Part model, mm, in its own coordinate system. Face numbers are marked on the shaded views. Coordinates: 2 decimals unless noted, no trailing zeros. Order: outer loops, then holes, each group sorted by start corner. A loop starts at its lowest first (then second) coordinate and runs counter-clockwise, first axis right, second up.
1) Cut at C-C (y = 6). Give the number of separate pieces and of enclosed holes in the cut face, and give its area (3 significant figures).
2) Pin check, flat tips, straight feed: pin 1 Ø1 at (y, z) = (33, 167.5) entering from -X; pin 2 Ø2 at (y, z) = (24, 180) entering from +X; pin 3 Ø4 at (y, z) = (36, 116) entering from -X; pin 4 Ø5 at (y, z) = (11.5, 154) entering from -X. Stop position of each tip, or through.
3) Cut at B-B (z = 101.6). List the corners of the cut face in (x, y).
4) Cut at A-A (x = -355.6). List the corners of the cut face in (y, z).
5) Wall check: L1, parallel to X at y = 38, z = 89; L2, parallel to Z at x = -100.5, y = 10; L3, parallel to X at y = 35.5, z = 87. Give the ranges that are in metal, low to high.
6) Cut at D-D (z = 152.4). List the corners of the cut face in (x, y), and give its area (3 significant figures).
7) Mould opens along Z. For the marked faces 1, 2, 3 and 4 say: +Z half, -Z half, draft (parallel to the pull), parting line (faces both ways), or undercut.
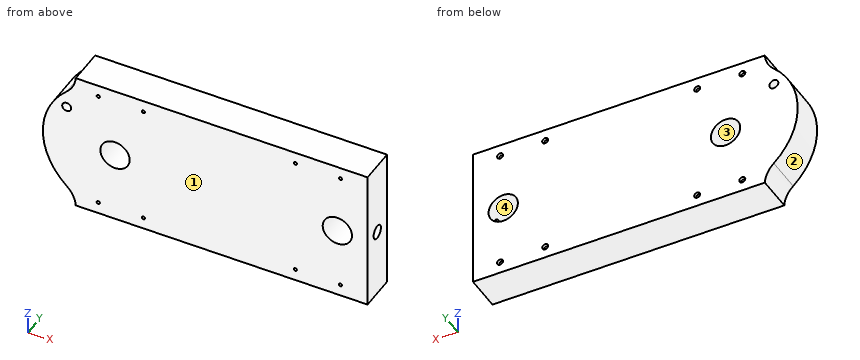
```python
from build123d import *

# Parameters (mm, degrees)
BOSS_EXTRUDE1_DEPTH                               = 50.8
CSK_FOR_8_FLAT_HEAD_MACHINE_SCREW_100_D           = 4.4958
CSK_FOR_8_FLAT_HEAD_MACHINE_SCREW_100_CSINK_D     = 8.4328
CSK_FOR_8_FLAT_HEAD_MACHINE_SCREW_100_CSINK_ANGLE = 82
MIRROR2_COPY_1_D                                  = 4.4958
MIRROR2_COPY_1_CSINK_D                            = 8.4328
MIRROR2_COPY_1_CSINK_ANGLE                        = 82
SKETCH14_R                                        = 6.35
CUT_EXTRUDE4_DEPTH                                = 503.89434278
SKETCH15_R                                        = 20.6375
CUT_EXTRUDE5_DEPTH                                = 503.89434278
SKETCH16_R                                        = 20.6375
CUT_EXTRUDE6_DEPTH                                = 503.89434278
F_5_8_0_75_DIAMETER_HOLE1_D                       = 19.05
F_5_8_0_75_DIAMETER_HOLE1_DEPTH                   = 32.961002604
F_5_8_0_75_DIAMETER_HOLE1_TIP                     = 5.723197396


with BuildPart() as part:
    # Sketch1 → Boss-Extrude1 (new body)
    with BuildSketch(Plane(origin=(0, 0, 0), x_dir=(1, 0, 0), z_dir=(0, 1, 0))):
        with BuildLine():
            Line((0, 0), (0, -203.2))
            Line((0, -203.2), (-410.920118429, -203.2))
            ThreePointArc((-410.920118429, -203.2), (-414.643880683, -188.956317144), (-423.489894398, -177.187844516))
            ThreePointArc((-423.489894398, -177.187844516), (-457.2, -101.6), (-423.489894398, -26.012155484))
            ThreePointArc((-423.489894398, -26.012155484), (-414.643880683, -14.243682856), (-410.920118429, 0))
            Line((-410.920118429, 0), (0, 0))
        make_face()
    extrude(amount=BOSS_EXTRUDE1_DEPTH)

    # CSK for #8 Flat Head Machine Screw (100)1 (through all)
    with Locations(Plane(origin=(0, 50.8, 0), x_dir=(1, 0, 0), z_dir=(0, 1, 0))):
        with Locations((-379.170118429, -186.3852), (-315.670118429, -186.3852)):
            csk_for_8_flat_head_machine_screw_100 = CounterSinkHole(CSK_FOR_8_FLAT_HEAD_MACHINE_SCREW_100_D / 2, CSK_FOR_8_FLAT_HEAD_MACHINE_SCREW_100_CSINK_D / 2, counter_sink_angle=CSK_FOR_8_FLAT_HEAD_MACHINE_SCREW_100_CSINK_ANGLE)

    # Mirror1: CSK for #8 Flat Head Machine Screw (100)1 across plane
    add(csk_for_8_flat_head_machine_screw_100.mirror(Plane.XY.offset(101.6)), mode=Mode.SUBTRACT)

    # Mirror2: CSK for #8 Flat Head Machine Screw (100)1 across plane
    add(csk_for_8_flat_head_machine_screw_100.mirror(Plane(origin=(-208.661, 0, 0), x_dir=(0, 0, 1), z_dir=(1, 0, 0))), mode=Mode.SUBTRACT)

    # Mirror2 copy 1 (through all)
    with Locations(Plane(origin=(-417.322, 50.8, 203.2), x_dir=(-1, 0, 0), z_dir=(0, 1, 0))):
        with Locations((-379.170118429, -186.3852), (-315.670118429, -186.3852)):
            CounterSinkHole(MIRROR2_COPY_1_D / 2, MIRROR2_COPY_1_CSINK_D / 2, counter_sink_angle=MIRROR2_COPY_1_CSINK_ANGLE)

    # Sketch14 → Cut-Extrude4 (cut, through all)
    with BuildSketch(Plane(origin=(0, 50.8, 0), x_dir=(1, 0, 0), z_dir=(0, 1, 0))):
        with Locations(Location((-423.620118429, -152.4, 0), (0, 0, 270))):
            Circle(SKETCH14_R)
    extrude(amount=-CUT_EXTRUDE4_DEPTH, mode=Mode.SUBTRACT)

    # Sketch15 → Cut-Extrude5 (cut, through all)
    with BuildSketch(Plane(origin=(0, 50.8, 0), x_dir=(1, 0, 0), z_dir=(0, 1, 0))):
        with Locations(Location((-355.6, -101.6, 0), (0, 0, 270))):
            Circle(SKETCH15_R)
    extrude(amount=-CUT_EXTRUDE5_DEPTH, mode=Mode.SUBTRACT)

    # Sketch16 → Cut-Extrude6 (cut, through all)
    with BuildSketch(Plane(origin=(0, 50.8, 0), x_dir=(1, 0, 0), z_dir=(0, 1, 0))):
        with Locations(Location((-42.545, -101.6, 0), (0, 0, 270))):
            Circle(SKETCH16_R)
    extrude(amount=-CUT_EXTRUDE6_DEPTH, mode=Mode.SUBTRACT)

    # 5/8 (0.75) Diameter Hole1
    with Locations(Plane(origin=(0, 0, 0), x_dir=(0, 0, -1), z_dir=(1, 0, 0))):
        with Locations((-97.7392, 25.4)):
            Hole(F_5_8_0_75_DIAMETER_HOLE1_D / 2, depth=F_5_8_0_75_DIAMETER_HOLE1_DEPTH)
            with Locations((0, 0, -(F_5_8_0_75_DIAMETER_HOLE1_DEPTH + F_5_8_0_75_DIAMETER_HOLE1_TIP / 2))):  # 118° drill point
                Cone(0, F_5_8_0_75_DIAMETER_HOLE1_D / 2, F_5_8_0_75_DIAMETER_HOLE1_TIP, mode=Mode.SUBTRACT)


solid = part.part
```
Geometry check:
1. separate pieces: 1
1. enclosed holes: 11
1. area: 86,200 mm2
2. pin 1: stops at x = -433.35
2. pin 2: stops at x = 0
2. pin 3: stops at x = -456.44
2. pin 4: stops at x = -444.1
3. outline: (-457.2, 0) - (-376.24, 0) - (-376.24, 50.8) - (-457.2, 50.8) - close; (-334.96, 0) - (-63.18, 0) - (-63.18, 50.8) - (-334.96, 50.8) - close; (-21.91, 0) - (0, 0) - (0, 16.69) - (-21.91, 16.69) - close; (-21.91, 34.11) - (0, 34.11) - (0, 50.8) - (-21.91, 50.8) - close
4. outline: (0, 0) - (50.8, 0) - (50.8, 80.96) - (0, 80.96) - close; (0, 122.24) - (50.8, 122.24) - (50.8, 203.2) - (0, 203.2) - close
5. L1: x = -456.42 to -371.94, -339.26 to -58.89, -26.2 to 0
5. L2: z = 0 to 14.88, 18.75 to 184.45, 188.32 to 203.2
5. L3: x = -456.15 to -370.19, -341.01 to -57.13, -27.96 to 0
6. outline: (-443.59, 0) - (-429.97, 0) - (-429.97, 50.8) - (-443.59, 50.8) - close; (-417.27, 0) - (0, 0) - (0, 50.8) - (-417.27, 50.8) - close
6. area: 21,900 mm2
7. face 1: draft
7. face 2: parting line
7. face 3: undercut
7. face 4: undercut
